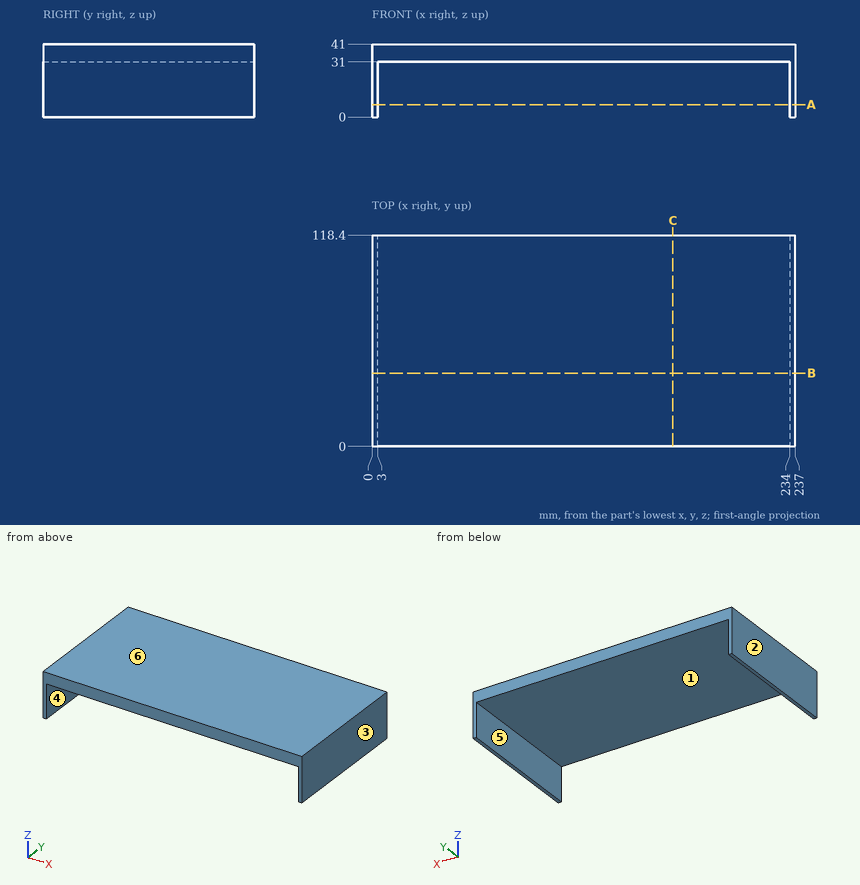
Study the drawing (mm; zero at the part's minimum x, y, z) and answer. A direction names the side the tool comes from. Round coordinates to 2 decimals unless told otherwise and drop trailing zeros. Write each loop counter-clockwise with the first axis right and the second up, starting at its lowest first coordinate (ties: lowest second). Pieces come first, ordered by that corner, then holes. Notation, with made-up numbers: (81, 41) -> (124, 41) arc R11 ccw to (124, 54) -> close; hole circle Ø6 at (43, 21.25). An arc over 180 degrees is marked (long way). Use CSV: the item, a comma, the result in double quotes. Start each with the question number.
(1) Section A-A on z = 7 is taken. Give the vertices of the cut face in (x, y).
(2) Consider L1, parallel to X at y = 26, z = 9.5; L2, parallel to Z at x = 56.5, y = 10. Determine where each line is inside the solid, lowest interval first. Write a range as from..to.
(3) Section C-C on x = 168.5 is taken. Give the vertices of the cut face in (y, z).
(4) This flat-tipped pin is pushed along its axis until it touches: pin 1 (10 mm diameter, centred on x = 107.5, z = 33, fed in from -Y). Where does it stop, or does it pass through?
(5) The mould has two halves that part along X. Classify the marked faces 1, 2, 3 and 4: released by +X, released by -X, zero draft, split by the parting line, or undercut.
(6) Which of the six approach directions +Z, -Z, +X, -X, +Y, -Y give full straight-line access (tool end or side, diameter ignored) to the marked faces 5 and 6?
(7) Section B-B on y = 41 is taken. Give the vertices of the cut face in (x, z), then the cut area to 3 significant figures.
A:
1,outline,"(0, 0) -> (3, 0) -> (3, 118.4) -> (0, 118.4) -> close; (234, 0) -> (237, 0) -> (237, 118.4) -> (234, 118.4) -> close"
2,L1,"x = 0..3, 234..237"
2,L2,"z = 31..41"
3,outline,"(0, 31) -> (118.4, 31) -> (118.4, 41) -> (0, 41) -> close"
4,pin 1,"stops at y = 0"
5,face 1,"undercut"
5,face 2,"released by -X"
5,face 3,"released by +X"
5,face 4,"undercut"
6,face 5,"-Z, +Y, -Y"
6,face 6,"+Z, +X, -X, +Y, -Y"
7,outline,"(0, 0) -> (3, 0) -> (3, 31) -> (234, 31) -> (234, 0) -> (237, 0) -> (237, 41) -> (0, 41) -> close"
7,area,"2,560 mm²"
